from build123d import *

# Parameters (mm, degrees)
SKETCH_1_W               = 65
SKETCH_1_H               = 45
EXTRUDE_1_DEPTH          = 28
SKETCH_2_W               = 46
SKETCH_2_H               = 24
CUT_EXTRUDE_1_DEPTH      = 39
FILLET_1_R               = 10
FILLET_2_R               = 10
FILLET_3_R               = 10
FILLET_4_R               = 10
SKETCH_9_W               = 5
SKETCH_9_H               = 34.070621565
CUT_EXTRUDE_2_DEPTH      = 1
CUT_EXTRUDE_2_DEPTH_BACK = 1
SKETCH_10_W              = 5
SKETCH_10_H              = 1
EXTRUDE_5_DEPTH          = 5
SKETCH_12_R              = 1.1
CUT_EXTRUDE_3_DEPTH      = 5
PATTERN_LINEAR_1_COUNT   = 2
PATTERN_LINEAR_1_PITCH   = 33
PATTERN_LINEAR_2_COUNT   = 2
PATTERN_LINEAR_2_PITCH   = 33


with BuildPart() as part:
    # 草圖1 → 填料-伸長1 (new body)
    with BuildSketch(Plane.XY):
        with Locations((-27.434655272, 0)):
            Rectangle(SKETCH_1_W, SKETCH_1_H)
    extrude(amount=EXTRUDE_1_DEPTH)

    # 草圖2 → 除料-伸長1 (cut)
    with BuildSketch(Plane.XY):
        with Locations((-27.434655272, 0)):
            Rectangle(SKETCH_2_W, SKETCH_2_H)
    extrude(amount=CUT_EXTRUDE_1_DEPTH, mode=Mode.SUBTRACT)

    # 圓角1
    fillet_1_edges = [part.edges().sort_by_distance(p)[0] for p in [
        (-59.934655272, -22.5, 14),
    ]]
    fillet(fillet_1_edges, radius=FILLET_1_R)

    # 圓角2
    fillet_2_edges = [part.edges().sort_by_distance(p)[0] for p in [
        (-59.934655272, 22.5, 14),
    ]]
    fillet(fillet_2_edges, radius=FILLET_2_R)

    # 圓角3
    fillet_3_edges = [part.edges().sort_by_distance(p)[0] for p in [
        (5.065344728, 22.5, 14),
    ]]
    fillet(fillet_3_edges, radius=FILLET_3_R)

    # 圓角4
    fillet_4_edges = [part.edges().sort_by_distance(p)[0] for p in [
        (5.065344728, -22.5, 14),
    ]]
    fillet(fillet_4_edges, radius=FILLET_4_R)

    # 草圖9 → 除料-伸長2 (cut, two sides)
    with BuildSketch(Plane(origin=(0, 0, 0), x_dir=(1, 0, 0), z_dir=(0, 1, 0))) as cut_extrude_2_sk:
        with Locations((2.565344728, -13.723230761)):
            Rectangle(SKETCH_9_W, SKETCH_9_H)
    extrude(amount=CUT_EXTRUDE_2_DEPTH, mode=Mode.SUBTRACT)
    extrude(cut_extrude_2_sk.sketch, amount=-CUT_EXTRUDE_2_DEPTH_BACK, mode=Mode.SUBTRACT)

    # 草圖10 → 填料-伸長5 (add)
    with BuildSketch(Plane.XY):
        with Locations((2.565344728, -1.5)):
            Rectangle(SKETCH_10_W, SKETCH_10_H)
        with Locations((2.565344728, 1.5)):
            Rectangle(SKETCH_10_W, SKETCH_10_H)
    extrude_5 = extrude(amount=-EXTRUDE_5_DEPTH)

    # 草圖12 → 除料-伸長3 (cut)
    with BuildSketch(Plane(origin=(0, -2, 0), x_dir=(-1, 0, 0), z_dir=(0, -1, 0))):
        with Locations((-2.565344728, 2.5)):
            Circle(SKETCH_12_R)
    cut_extrude_3 = extrude(amount=-CUT_EXTRUDE_3_DEPTH, mode=Mode.SUBTRACT)

    # 直線複製排列1: 填料-伸長5 ×2
    with Locations(*[(0, 0, i * PATTERN_LINEAR_1_PITCH) for i in range(1, PATTERN_LINEAR_1_COUNT)]):
        add(extrude_5)

    # 直線複製排列2: 除料-伸長3 ×2
    with Locations(*[(0, 0, i * PATTERN_LINEAR_2_PITCH) for i in range(1, PATTERN_LINEAR_2_COUNT)]):
        add(cut_extrude_3, mode=Mode.SUBTRACT)


solid = part.part
Source: CAD feature listing. Evaluate the final solid. Frame: model axes, mm. A direction names the side the tool comes from. Round coordinates to 2 decimals unless told otherwise and drop trailing zeros. Write each loop counter-clockwise with the first axis right and the second up, starting at its lowest first coordinate (ties: lowest second). Pieces come first, ordered by that corner, then holes. Notation, with made-up numbers: M 47.5,-6 L 83.5,-6 A25 cw 83.5,22 Z; hole C 81.25,18 d5. An arc over 180 degrees is marked long. One line per item, written item: value. Start each with the question number.
Item 1: Section query A-A (x = -47). Return the cut outline in (y, z).
Item 2: Section query C-C (z = 8.5). Return the cut outline in (x, y), plus the area to 3 significant figures.
Item 3: Set-up query: faces 4 (the flat face through (0.065, 0, 14)), 5 (the flat face through (3, -2, 32)), 6 (the flat face through (-28, -22.5, 14)), 7 (the flat face through (-28, -12, 14)), 8 (the flat face through (3, 2, -1)). Return all of +Z, -Z, +X, -X, +Y, -Y with unobstructed straight access to the full face (end or side cutting, diameter ignored); none if empty.
Item 4: Ray query, L1, parallel to X at y = -1.25, z = -2.5; L2, parallel to Y at x = -41, z = 7.5; L3, parallel to X at y = -9.5, z = 0.5. Return the intervals inside material, ascending. Write a range as from..to.
Item 5: Mould query, pull axis X, two halves, no side actions, for faces 1 (the flat face through (-28, 22.5, 14)), 2 (the cylindrical face through (2.804, 1.493, 31.574)), 3 (the flat face through (-59.935, 0, 14)). Classes: pulls with the +X half, pulls with the -X half, needs draft (parallel to the pull), parting line crosses it, or undercut.
Item 6: Pin query (flat end, axial travel): pin 1 (3 mm diameter, centred on x = -3.5, y = 4.5, fed in from -Z); pin 2 (10 mm diameter, centred on x = -42, y = -3, fed in from +Z); pin 3 (12 mm diameter, centred on x = -3.5, y = 17, fed in from +Z); pin 4 (2.5 mm diameter, centred on x = 2.57, z = 30.5, fed in from +Y). Return the tip coordinate at first contact, or that it passes through.
Item 7: Section query B-B (z = -2.5). Return the cut outline in (x, y), plus the area to 3 significant figures.
Item 8: Section query D-D (y = -4.5). Return the cut outline in (x, z), plus the area to 3 significant figures.
Result set:
1. outline: M -22.5,0 L -12,0 L -12,28 L -22.5,28 Z; M 12,0 L 22.5,0 L 22.5,28 L 12,28 Z
2. outline: M -59.93,-12.5 A10 ccw -49.93,-22.5 L -4.93,-22.5 A10 ccw 5.07,-12.5 L 5.07,-1 L 0.07,-1 L 0.07,1 L 5.07,1 L 5.07,12.5 A10 ccw -4.93,22.5 L -49.93,22.5 A10 ccw -59.93,12.5 Z; hole M -50.43,-12 L -4.43,-12 L -4.43,12 L -50.43,12 Z
2. area: 1,730 mm²
3. face 4: +Z, -Z, +X
3. face 5: +Z, +X, -X, -Y
3. face 6: +Z, -Z, +X, -X, -Y
3. face 7: +Z, -Z
3. face 8: -Z, +X, -X, +Y
4. L1: x = 0.07..1.47, 3.67..5.07
4. L2: y = -22.5..-12, 12..22.5
4. L3: x = -59.93..-50.43, -4.43..5.07
5. face 1: needs draft
5. face 2: undercut
5. face 3: pulls with the -X half
6. pin 1: stops at z = 0
6. pin 2: passes through
6. pin 3: stops at z = 28
6. pin 4: stops at y = 2
7. outline: M 0.07,-2 L 1.47,-2 L 1.47,-1 L 0.07,-1 Z; M 0.07,1 L 1.47,1 L 1.47,2 L 0.07,2 Z; M 3.67,-2 L 5.07,-2 L 5.07,-1 L 3.67,-1 Z; M 3.67,1 L 5.07,1 L 5.07,2 L 3.67,2 Z
7. area: 5.60 mm²
8. outline: M -59.93,0 L -50.43,0 L -50.43,28 L -59.93,28 Z; M -4.43,0 L 5.07,0 L 5.07,28 L -4.43,28 Z
8. area: 532 mm²
